Design review of the part shown in the three views and the two pictorial views. Dimensions are in mm from the part's minimum x, y and z. A direction names the side the tool comes from. Coordinates: 2 decimals unless noted, no trailing zeros. Order: outer loops, then holes, each group sorted by start corner. A loop starts at its lowest first (then second) coordinate and runs counter-clockwise, first axis right, second up. Notation, with made-up numbers: M -28.75,52 L 25.25,52 A9 cw 25.25,63 Z; hole C -25,58 d1. An arc over 180 degrees is marked long. Use CSV: the item, a comma, the result in double quotes.
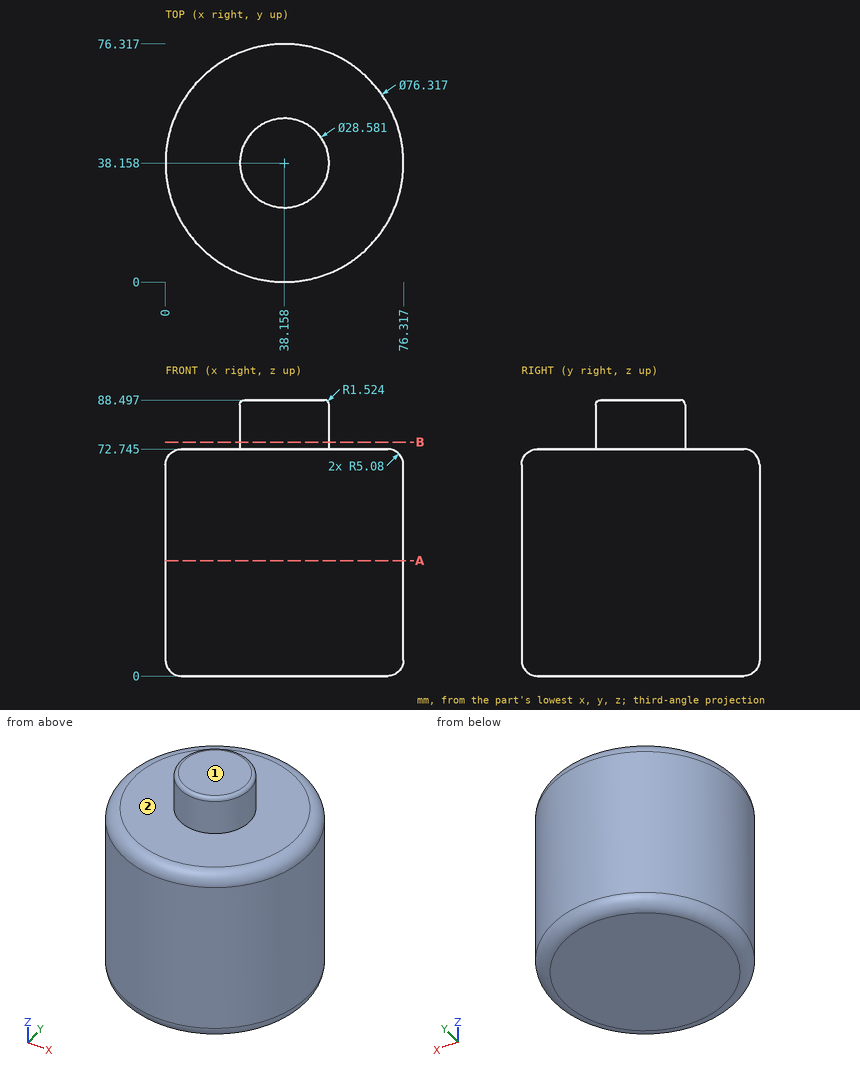
(1) For the marked faces 1 and 2, list the 3-axis set-ups (+Z, -Z, +X, -X, +Y, -Y) from which the entire face can be reached by the end or side of a thin tool; tool diameter is ignored.
The answers:
face 1,"+Z, +X, -X, +Y, -Y"
face 2,"+Z"
(2) Add section B-B on z = 75. State the section outline as (x, y) points.
The answers:
outline,"C 38.16,38.16 d28.58"
(3) Wall thickness on probe 1 along Z at (x, y) = (61, 23) (1 decimal); probe 2 along X at (y, z) = (45, 44); probe 3 along Y at (x, z) = (10, 14) (1 decimal): over which ranges is each line inside the solid? List them lowest first.
The answers:
probe 1,"z = 0 to 72.7"
probe 2,"x = 0.62 to 75.7"
probe 3,"y = 12.4 to 63.9"
(4) Add section A-A on z = 37. State the section outline as (x, y) points.
The answers:
outline,"C 38.16,38.16 d76.32"
(5) Clearance check with flat-ended pins moving along their axes: P1, Ø1, axis at x = 18.5, z = 30.5, coming from the +Y side; P2, Ø6, axis at y = 28, z = 54.5, coming from the -X side; P3, Ø8, axis at x = 49.5, z = 15.5, coming from the +Y side. State where each tip first meets the part, or that it passes through.
The answers:
P1,"stops at y = 71.16"
P2,"stops at x = 0.68"
P3,"stops at y = 75.6"
